The listing builds one solid part. Answer for the finished solid, in the listing's coordinates (mm). A direction names the side the tool comes from. Round coordinates to 2 decimals unless told otherwise and drop trailing zeros. Write each loop counter-clockwise with the first axis right and the second up, starting at its lowest first coordinate (ties: lowest second). Pieces come first, ordered by that corner, then holes. Notation, with made-up numbers: (40, 80.25) - (60, 80.25) arc R17 ccw to (60, 90.25) - close; hole circle Ø5 at (-27, 3). An arc over 180 degrees is marked (long way). Answer in a Markdown table with one row per item.
from build123d import *

# Parameters (mm, degrees)
SKETCH1_R           = 35
SKETCH1_R_2         = 3
BOSS_EXTRUDE1_DEPTH = 12.5
SKETCH2_R           = 40
SKETCH2_R_2         = 35
BOSS_EXTRUDE2_DEPTH = 15


with BuildPart() as part:
    # Sketch1 → Boss-Extrude1 (new, symmetric)
    with BuildSketch(Plane(origin=(0, 0, 0), x_dir=(0, 0, -1), z_dir=(1, 0, 0))):
        Circle(SKETCH1_R)
        Circle(SKETCH1_R_2, mode=Mode.SUBTRACT)
        with BuildLine():
            Line((0, 28), (0, 8))
            ThreePointArc((0, 8), (2.736161147, 7.517540966), (5.142300877, 6.128355545))
            Line((5.142300877, 6.128355545), (17.998053071, 21.449244407))
            ThreePointArc((17.998053071, 21.449244407), (9.576564013, 26.311393382), (0, 28))
        make_face(mode=Mode.SUBTRACT)
        with BuildLine():
            Line((26.629582456, 8.652475842), (7.60845213, 2.472135955))
            ThreePointArc((7.60845213, 2.472135955), (7.995126616, -0.279195974), (7.417470837, -2.996852747))
            Line((7.417470837, -2.996852747), (25.961147928, -10.488984616))
            ThreePointArc((25.961147928, -10.488984616), (27.982943157, -0.977185908), (26.629582456, 8.652475842))
        make_face(mode=Mode.SUBTRACT)
        with BuildLine():
            Line((16.457987064, -22.652475842), (4.702282018, -6.472135955))
            ThreePointArc((4.702282018, -6.472135955), (2.205098847, -7.690093568), (-0.55805179, -7.980512402))
            Line((-0.55805179, -7.980512402), (-1.953181265, -27.931793407))
            ThreePointArc((-1.953181265, -27.931793407), (7.717845963, -26.915327486), (16.457987064, -22.652475842))
        make_face(mode=Mode.SUBTRACT)
        with BuildLine():
            Line((-16.457987064, -22.652475842), (-4.702282018, -6.472135955))
            ThreePointArc((-4.702282018, -6.472135955), (-6.63230058, -4.473543228), (-7.76236581, -1.935375165))
            Line((-7.76236581, -1.935375165), (-27.168280336, -6.773813077))
            ThreePointArc((-27.168280336, -6.773813077), (-23.213052032, -15.657401297), (-16.457987064, -22.652475842))
        make_face(mode=Mode.SUBTRACT)
        with BuildLine():
            Line((-26.629582456, 8.652475842), (-7.60845213, 2.472135955))
            ThreePointArc((-7.60845213, 2.472135955), (-6.304086029, 4.925291803), (-4.239354114, 6.784384769))
            Line((-4.239354114, 6.784384769), (-14.837739399, 23.745346692))
            ThreePointArc((-14.837739399, 23.745346692), (-22.064301101, 17.238521309), (-26.629582456, 8.652475842))
        make_face(mode=Mode.SUBTRACT)
    extrude(amount=BOSS_EXTRUDE1_DEPTH, both=True)

    # Sketch2 → Boss-Extrude2 (add, symmetric)
    with BuildSketch(Plane(origin=(0, 0, 0), x_dir=(0, 0, -1), z_dir=(1, 0, 0))):
        Circle(SKETCH2_R)
        Circle(SKETCH2_R_2, mode=Mode.SUBTRACT)
    extrude(amount=BOSS_EXTRUDE2_DEPTH, both=True)


solid = part.part
(1) For faces 1 (the cylindrical face through (14, -21, 28)), 2 (the flat face through (0.18, -4.32, 17.33)), determine the directions among +Z, -Z, +X, -X, +Y, -Y from which every point of the face is accessible in a straight line to the end or side of a thin tool.
Checked values:
| item | result |
|---|---|
| face 1 | +X |
| face 2 | +X, -X |
(2) Section C-C (z = -9) is taken. Give the vertices of the cut face in (x, y).
Checked values:
| item | result |
|---|---|
| outline | (-15, -38.97) - (15, -38.97) - (15, -33.82) - (12.5, -33.82) - (12.5, -26.51) - (-12.5, -26.51) - (-12.5, -33.82) - (-15, -33.82) - close; (-15, 33.82) - (-12.5, 33.82) - (-12.5, 26.51) - (12.5, 26.51) - (12.5, 33.82) - (15, 33.82) - (15, 38.97) - (-15, 38.97) - close; (-12.5, -12.39) - (12.5, -12.39) - (12.5, -3.64) - (-12.5, -3.64) - close; (-12.5, 2.92) - (12.5, 2.92) - (12.5, 10.73) - (-12.5, 10.73) - close |
(3) Flat-ended cylindrical pins translate along their axes: pin 1 (2 mm diameter, centred on y = -22, z = -16, fed in from +X); pin 2 (5.5 mm diameter, centred on y = 0, z = 0, fed in from +X); pin 3 (3 mm diameter, centred on x = -5.5, y = -13, fed in from -Z); pin 4 (4 mm diameter, centred on x = -7, z = -0.5, fed in from +Y). Find the tip coordinate at first contact, or state that the pin passes through.
Checked values:
| item | result |
|---|---|
| pin 1 | stops at x = 12.5 |
| pin 2 | passes through |
| pin 3 | stops at z = -38.31 |
| pin 4 | stops at y = 40 |
(4) Find the intervals of material crossed by line 1 (Z direction, x = -11.5, y = -12); line 2 (Y direction, x = 1.5, z = 12); line 3 (Z direction, x = -4.25, y = -13.5), in increasing order.
Checked values:
| item | result |
|---|---|
| line 1 | z = -38.16 to -8.72, 0.84 to 8.72, 25.3 to 38.16 |
| line 2 | y = -38.16 to -16.52, -2.99 to 3.9, 19.2 to 38.16 |
| line 3 | z = -37.65 to -9.81, 0.94 to 9.81, 24.53 to 37.65 |
(5) Section A-A (y = 0) is taken. Give the vertices of the cut face in (x, z).
Checked values:
| item | result |
|---|---|
| outline | (-15, -40) - (15, -40) - (15, -35) - (12.5, -35) - (12.5, -28) - (-12.5, -28) - (-12.5, -35) - (-15, -35) - close; (-15, 35) - (-12.5, 35) - (-12.5, 3) - (12.5, 3) - (12.5, 35) - (15, 35) - (15, 40) - (-15, 40) - close; (-12.5, -8) - (12.5, -8) - (12.5, -3) - (-12.5, -3) - close |
(6) For a pull along Y with two mould halves and no side action, classify faces 3 (the cylindrical face through (0.175, -4.506, 6.61)), 4 (the cylindrical face through (-14, -21, 28)), 5 (the cylindrical face through (0.21, -39.05, 8.67)), 6 (the flat face through (15, -35.4, 0.2)) as pulls with the +Y half, pulls with the -Y half, needs draft (parallel to the pull), parting line crosses it, or undercut.
Checked values:
| item | result |
|---|---|
| face 3 | undercut |
| face 4 | undercut |
| face 5 | parting line crosses it |
| face 6 | needs draft |
(7) Section B-B (x = -10) is taken. Give the vertices of the cut face in (y, z).
Checked values:
| item | result |
|---|---|
| outline | circle Ø80 at (0, 0); hole (-27.93, 1.95) arc R28 ccw to (-22.65, -16.46) - (-6.47, -4.7) arc R8 cw to (-7.98, 0.56) - close; hole (-22.65, 16.46) - (-6.47, 4.7) arc R8 cw to (-1.94, 7.76) - (-6.77, 27.17) arc R28 ccw to start; hole (-10.49, -25.96) arc R28 ccw to (8.65, -26.63) - (2.47, -7.61) arc R8 cw to (-3, -7.42) - close; hole circle Ø6 at (0, 0); hole (2.47, 7.61) arc R8 cw to (6.78, 4.24) - (23.75, 14.84) arc R28 ccw to (8.65, 26.63) - close; hole (6.13, -5.14) - (21.45, -18) arc R28 ccw to (28, 0) - (8, 0) arc R8 cw to start |
(8) Section D-D (y = 25.5) is taken. Give the vertices of the cut face in (x, z).
Checked values:
| item | result |
|---|---|
| outline | (-15, -30.82) - (15, -30.82) - (15, -23.97) - (12.5, -23.97) - (12.5, -11.57) - (-12.5, -11.57) - (-12.5, -23.97) - (-15, -23.97) - close; (-15, 23.97) - (-12.5, 23.97) - (-12.5, 0) - (12.5, 0) - (12.5, 23.97) - (15, 23.97) - (15, 30.82) - (-15, 30.82) - close |
